For this review, take the finished solid that the model builds, in its own axes (mm). Face numbers are marked on the shaded views. A direction names the side the tool comes from. Round coordinates to 2 decimals unless told otherwise and drop trailing zeros. Write each loop counter-clockwise with the first axis right and the second up, starting at its lowest first coordinate (ties: lowest second). Pieces come first, ordered by that corner, then holes. Notation, with made-up numbers: (-25, 69) -> (-8, 69) arc R11 cw to (-8, 90) -> close; hole circle Ø8 at (79, 78). An arc over 180 degrees is marked (long way). Answer as CSV lines item,"result". Start each with the question number.
Item 1: Wall thickness on probe 1 along Z at (x, y) = (-5.5, -17); probe 2 along Z at (x, y) = (29.5, 1); probe 3 along X at (y, z) = (-2.5, 6): over which ranges is each line inside the solid? List them lowest first. Write a range as from..to.
Item 2: Take a section at A-A on x = 34. Give the boundary of the cut face in (y, z).
Item 3: Take a section at B-B on z = 16. Give the boundary of the cut face in (x, y), then the cut area to 3 significant figures.
Item 4: Mouldability with a two-part tool opening along Z and no side actions: class the marked faces 4, 5, 6 and 7 as +Z half, -Z half, draft (parallel to the pull), parting line (faces both ways), or undercut.
Item 5: Take a section at D-D on y = 15.5. Give the boundary of the cut face in (x, z), then the cut area to 3 significant figures.
Item 6: For pin 1 Ø12 at (x, y) = (12.5, 7.5) entering from -Z; pin 2 Ø22 at (x, y) = (13, -14) entering from -Z; pin 3 Ø8 at (x, z) = (-14, 3.5) entering from -Y, all flat-tipped, find the tip position at first contact; note any pin that passes through.
Item 7: Machinability: for the marked faces 1, 2 and 3, which of the approach directions +Z, -Z, +X, -X, +Y, -Y give a long, thin tool a straight path to every point of the face, cutting with its end or side? Answer none if there is none.
Item 8: Take a section at C-C on x = 6. Give the boundary of the cut face in (y, z).
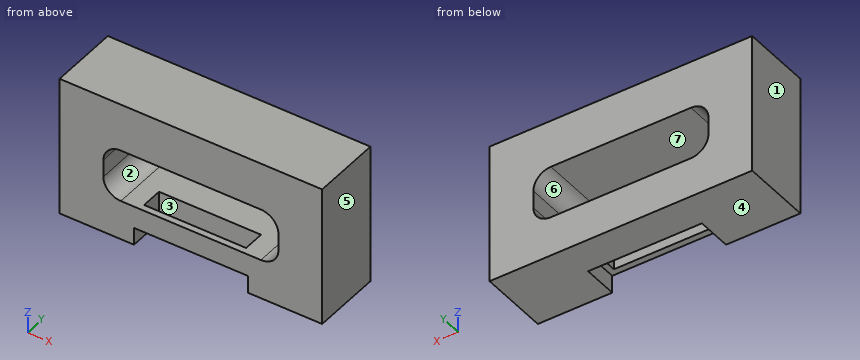
```python
from build123d import *

# Parameters (mm, degrees)
F0_W     = 150
F0_H     = 40
F1_DEPTH = 80
F2_W     = 65
F2_H     = 20
F3_DEPTH = 10
F5_DEPTH = 264.4
F6_W     = 58.287583
F6_H     = 12.372349
F7_DEPTH = 25


with BuildPart() as f1:
    # F0 (on Top) → F1 (new body)
    with BuildSketch(Plane.XY):
        Rectangle(F0_W, F0_H)
    extrude(amount=F1_DEPTH)

    # F2 (on face) → F3 (cut)
    with BuildSketch(Plane(origin=(0, 0, 0), x_dir=(1, 0, 0), z_dir=(0, 0, -1))):
        with Locations((0, 10)):
            Rectangle(F2_W, F2_H)
    extrude(amount=-F3_DEPTH, mode=Mode.SUBTRACT)

    # F4 (on face) → F5 (cut)
    with BuildSketch(Plane.XZ.offset(20)):
        with BuildLine():
            Line((-40, 22.681816), (40, 22.681816))
            ThreePointArc((40, 22.681816), (47.071068, 25.610749), (50, 32.681816))
            Line((50, 32.681816), (50, 42.681816))
            ThreePointArc((50, 42.681816), (47.071068, 49.752884), (40, 52.681816))
            Line((40, 52.681816), (-40, 52.681816))
            ThreePointArc((-40, 52.681816), (-47.071068, 49.752884), (-50, 42.681816))
            Line((-50, 42.681816), (-50, 32.681816))
            ThreePointArc((-50, 32.681816), (-47.071068, 25.610749), (-40, 22.681816))
        make_face()
    extrude(amount=-F5_DEPTH, mode=Mode.SUBTRACT)

    # F6 (on face) → F7 (cut)
    with BuildSketch(Plane(origin=(0, 0, 10), x_dir=(1, 0, 0), z_dir=(0, 0, -1))):
        with Locations((-0.142549, 10.109945)):
            Rectangle(F6_W, F6_H)
    extrude(amount=-F7_DEPTH, mode=Mode.SUBTRACT)


solid = f1.part
```
Output values:
1,probe 1,"z = 10..22.68, 52.68..80"
1,probe 2,"z = 0..22.68, 52.68..80"
1,probe 3,"x = -75..-32.5, 32.5..75"
2,outline,"(-20, 0) -> (20, 0) -> (20, 22.68) -> (-20, 22.68) -> close; (-20, 52.68) -> (20, 52.68) -> (20, 80) -> (-20, 80) -> close"
3,outline,"(-75, -20) -> (75, -20) -> (75, 20) -> (-75, 20) -> close; hole (-29.29, -16.3) -> (29, -16.3) -> (29, -3.92) -> (-29.29, -3.92) -> close"
3,area,"5,280 mm^2"
4,face 4,"-Z half"
4,face 5,"draft"
4,face 6,"undercut"
4,face 7,"undercut"
5,outline,"(-75, 0) -> (75, 0) -> (75, 80) -> (-75, 80) -> close; hole (-50, 32.68) arc R10 ccw to (-40, 22.68) -> (40, 22.68) arc R10 ccw to (50, 32.68) -> (50, 42.68) arc R10 ccw to (40, 52.68) -> (-40, 52.68) arc R10 ccw to (-50, 42.68) -> close"
5,area,"9,090 mm^2"
6,pin 1,"stops at z = 0"
6,pin 2,"stops at z = 10"
6,pin 3,"stops at y = 0"
7,face 1,"+Z, -Z, -X, +Y, -Y"
7,face 2,"+Y, -Y"
7,face 3,"-Z"
8,outline,"(-20, 10) -> (-16.3, 10) -> (-16.3, 22.68) -> (-20, 22.68) -> close; (-20, 52.68) -> (20, 52.68) -> (20, 80) -> (-20, 80) -> close; (-3.92, 10) -> (0, 10) -> (0, 0) -> (20, 0) -> (20, 22.68) -> (-3.92, 22.68) -> close"
